from build123d import *

# Parameters (mm, degrees)
EXTRUDE1_DEPTH = 3.175
SKETCH5_R      = 4.899523771
EXTRUDE2_DEPTH = 6.9215


with BuildPart() as part:
    # Sketch1 → Extrude1 (new body)
    with BuildSketch(Plane(origin=(0, 0, 0), x_dir=(1, 0, 0), z_dir=(0, 1, 0))):
        Polygon((131.293364516, 0), (137.643364516, 6.35), (137.643364516, 74.305125285), (131.293364516, 80.655125285), (6.35, 80.655125285), (0, 74.305125285), (0, 6.35), (6.35, 0), align=None)
    extrude(amount=-EXTRUDE1_DEPTH)

    # Sketch3 → Revolve1 (revolve)
    with BuildSketch(Plane.XY.offset(-19.05), mode=Mode.PRIVATE) as revolve1_sk:
        with BuildLine():
            Line((25.4, 0), (33.952460507, 0))
            Line((33.952460507, 0), (33.952460507, 0.90459086))
            ThreePointArc((33.952460507, 0.90459086), (33.87806563, 1.084195983), (33.698460507, 1.15859086))
            Line((33.698460507, 1.15859086), (32.962971663, 1.15859086))
            ThreePointArc((32.962971663, 1.15859086), (32.792104444, 1.224653653), (32.710118846, 1.388477524))
            ThreePointArc((32.710118846, 1.388477524), (32.305713436, 2.5146954), (31.411407987, 3.309760306))
            ThreePointArc((31.411407987, 3.309760306), (30.665271183, 3.28370412), (30.299523771, 2.632837093))
            Line((30.299523771, 2.632837093), (30.299523771, 1.803708053))
            Line((30.299523771, 1.803708053), (25.4, 1.803708053))
            Line((25.4, 1.803708053), (25.4, 0))
        make_face()
    revolve(revolve1_sk.sketch.rotate(Axis((25.4, 0, -19.05), (0, 1, 0)), 90), axis=Axis((25.4, 0, -19.05), (0, 1, 0)))

    # Sketch5 → Extrude2 (cut, symmetric)
    with BuildSketch(Plane(origin=(0, 0, 0), x_dir=(1, 0, 0), z_dir=(0, 1, 0))):
        with Locations(Location((25.4, 19.05, 0), (0, 0, 90))):
            Circle(SKETCH5_R)
    extrude(amount=EXTRUDE2_DEPTH, both=True, mode=Mode.SUBTRACT)


solid = part.part
Could you check a few things on this model? Use its own coordinates, in mm. A direction names the side the tool comes from. Coordinates: 2 decimals unless noted, no trailing zeros. Loops run counter-clockwise (first coordinate to the right, second up) from the corner with the lowest first, then second, coordinate; pieces in that order, holes last.
1. I need wall thicknesses on L1, parallel to X at y = 0.35, z = -19.05; L2, parallel to Z at x = 25.4, y = -0.95; L3, parallel to Z at x = 25.4, y = 0.7. Which ranges of each line are inside material? Lowest first, please.
2. Imagine slicing it at B-B (z = -19.05). Please give me the cut outline in (x, y) (3 decimals), and give its area (3 significant figures).
3. For faces 4 (the face through (68, -3.175, -41)), 5 (the face through (33, 1.159, -17)), which set-ups out of +Z, -Z, +X, -X, +Y, -Y let a thin tool reach every point of the face, with its end or its side?
4. For P1, Ø1.5, axis at x = 63.5, y = -1.5, coming from the +Z side; P2, Ø3, axis at x = 77, z = -36.5, coming from the +Y side, each with a flat end and sliding along its axis, tell me the tip position at first contact or that it passes through.
5. Imagine slicing it at A-A (x = 25.4). Please give me the cut outline in (y, z) (3 decimals).
6. We'd pull the mould along Z, two halves only. Please class faces 1 (the face through (137.643, -2, -40)), 2 (the face through (22.09, -0.23, -15.44)), 3 (the face through (3.219, -1.565, -77.525)): released by +Z, released by -Z, zero draft, split by the parting line, or undercut.
7. Imagine slicing it at C-C (z = -33). Please give me the cut outline in (x, y) (3 decimals).
Computed values:
1. L1: x = 16.85 to 20.5, 30.3 to 33.95
1. L2: z = -80.66 to -23.95, -14.15 to 0
1. L3: z = -27.6 to -23.95, -14.15 to -10.5
2. outline: (0, -3.175) - (20.5, -3.175) - (20.5, 2.633) arc R0.762 ccw to (19.389, 3.31) arc R2.422 ccw to (18.09, 1.388) arc R0.254 cw to (17.837, 1.159) - (17.102, 1.159) arc R0.254 ccw to (16.848, 0.905) - (16.848, 0) - (0, 0) - close; (30.3, -3.175) - (137.643, -3.175) - (137.643, 0) - (33.952, 0) - (33.952, 0.905) arc R0.254 ccw to (33.698, 1.159) - (32.963, 1.159) arc R0.254 cw to (32.71, 1.388) arc R2.422 ccw to (31.411, 3.31) arc R0.762 ccw to (30.3, 2.633) - close
2. area: 423 mm2
3. face 4: +Z, -Z, +X, -X, -Y
3. face 5: +Y
4. P1: stops at z = 0
4. P2: stops at y = 0
5. outline: (-3.175, -80.655) - (0, -80.655) - (0, -27.602) - (0.905, -27.602) arc R0.254 ccw to (1.159, -27.348) - (1.159, -26.613) arc R0.254 cw to (1.388, -26.36) arc R2.422 ccw to (3.31, -25.061) arc R0.762 ccw to (2.633, -23.95) - (-3.175, -23.95) - close; (-3.175, -14.15) - (2.633, -14.15) arc R0.762 ccw to (3.31, -13.039) arc R2.422 ccw to (1.388, -11.74) arc R0.254 cw to (1.159, -11.487) - (1.159, -10.752) arc R0.254 ccw to (0.905, -10.498) - (0, -10.498) - (0, 0) - (-3.175, 0) - close
6. face 1: zero draft
6. face 2: undercut
6. face 3: released by -Z
7. outline: (0, -3.175) - (137.643, -3.175) - (137.643, 0) - (0, 0) - close
